Job drawing, mm, ordinate dimensions from the low corner. One solid piece. Coordinates: 2 decimals unless noted, no trailing zeros. Use a Markdown table: item, result. Add a question column.
1) Wall check: L1, parallel to Y at x = 9, z = 7.25; L2, parallel to Y at x = 3.5, z = 5.5. Give the ranges that are in metal, low to high. Write a range as [from, to].
2) Drop a flat-ended pin along its axis: P1, Ø0.5, axis at x = 1, y = 2, coming from the +Z side. Give the stop position or say it passes through.
3) Saw through at A-A on z = 5.75. Count the separate pieces of the cut face and the enclosed holes in it, then the cut area to 3 significant figures.
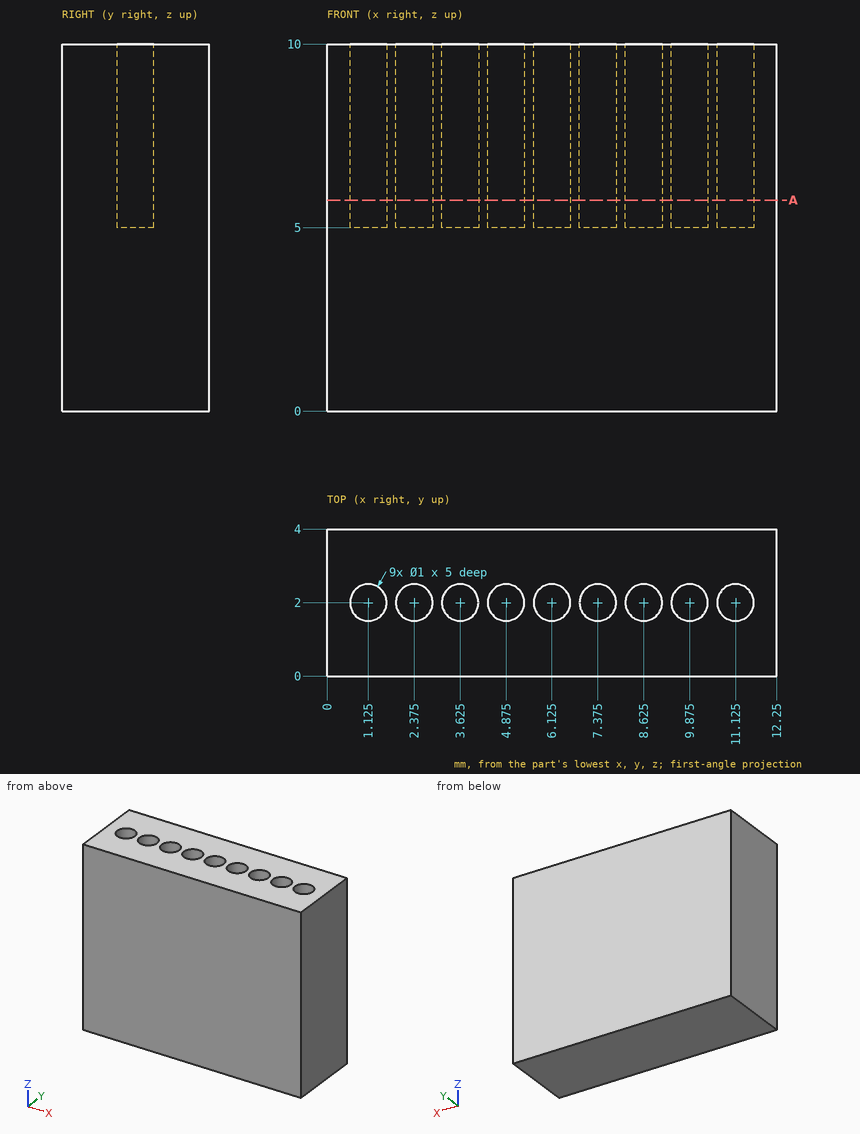
Results are:
| question | item | result |
|---|---|---|
| 1 | L1 | [0, 1.67], [2.33, 4] |
| 1 | L2 | [0, 1.52], [2.48, 4] |
| 2 | P1 | z = 5 |
| 3 | separate pieces | 1 |
| 3 | enclosed holes | 9 |
| 3 | area | 41.9 mm2 |
